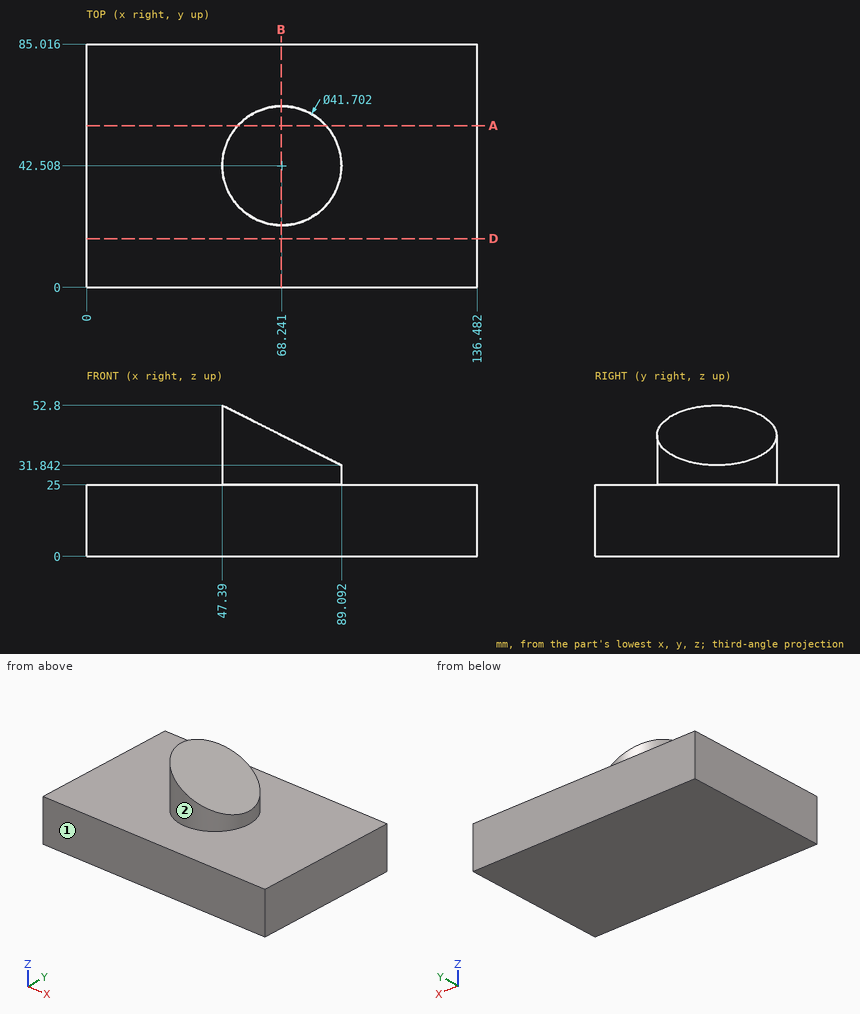
The drawing under review shows one solid part. Ordinate dimensions are in mm from its lowest x, y, z. A direction names the side the tool comes from. Round coordinates to 2 decimals unless told otherwise and drop trailing zeros. Loops run counter-clockwise (first coordinate to the right, second up) from the corner with the lowest first, then second, coordinate; pieces in that order, holes last. Notation, with made-up numbers: (-34, 11.25) - (20, 11.25) arc R10 cw to (20, 27.25) - close; hole circle Ø1 at (-21.75, 70.5). An arc over 180 degrees is marked (long way). One line per item, written item: value. Start each with the question number.
1) Consider section A-A on y = 56.5. Give the boundary of the cut face in (x, z), then the cut area to 3 significant figures.
2) Consider section D-D on y = 17. Give the boundary of the cut face in (x, z), then the cut area to 3 significant figures.
3) Insertion check: pin 1 Ø10 at (x, y) = (53.5, 10.5) entering from +Z. The pin has a flat end and moves straight along its axis. Give the tip position at first contact, or say it passes through.
4) Consider section B-B on x = 68. Give the boundary of the cut face in (y, z).
5) To check wall thickness, follow L1, parallel to Z at x = 51, y = 22; L2, parallel to X at y = 52, z = 42 (1 decimal); L3, parallel to X at y = 36.5, z = 49.5 (1 decimal). State the ranges of each line that lie inside material, in increasing order. Write a range as from..to.
6) For the marked faces 1 and 2, list the 3-axis set-ups (+Z, -Z, +X, -X, +Y, -Y) from which the entire face can be reached by the end or side of a thin tool; tool diameter is ignored.
Reported:
1. outline: (0, 0) - (136.48, 0) - (136.48, 25) - (83.7, 25) - (83.7, 34.55) - (52.78, 50.09) - (52.78, 25) - (0, 25) - close
1. area: 3,950 mm^2
2. outline: (0, 0) - (136.48, 0) - (136.48, 25) - (0, 25) - close
2. area: 3,410 mm^2
3. pin 1: stops at z = 25
4. outline: (0, 0) - (85.02, 0) - (85.02, 25) - (63.36, 25) - (63.36, 42.44) - (21.66, 42.44) - (21.66, 25) - (0, 25) - close
5. L1: z = 0..25
5. L2: x = 49.7..68.9
5. L3: x = 48.3..54
6. face 1: +Z, -Z, +X, -X, -Y
6. face 2: +Z
